Input: dimensioned drawing with shaded views. Units: mm. Origin: part minimum x, y, z. A direction names the side the tool comes from. Round coordinates to 2 decimals unless told otherwise and drop trailing zeros. Order: outer loops, then holes, each group sorted by start corner. A loop starts at its lowest first (then second) coordinate and runs counter-clockwise, first axis right, second up. Notation, with made-up numbers: M 47.5,45 L 98.5,45 A27 ccw 98.5,78 Z; hole C 1,85 d6. An arc over 180 degrees is marked long. Put each result on its own line as item: value. Start each with the question number.
1) Section B-B, the plane y = 0.55. Return loops of the section in (x, z), then the cut area to 3 significant figures.
2) Section C-C, the plane x = 12.25. Return loops of the section in (y, z), then the cut area to 3 significant figures.
3) Section A-A, the plane z = 3.75. Return loops of the section in (x, y).
4) Material intervals for probe 1 along X at (y, z) = (1.2, 4); probe 2 along Z at (x, y) = (5.5, 1.9); probe 3 along X at (y, z) = (2.25, 6.25), sorted ascending. Write a range as [from, to].
5) Section D-D, the plane z = 6.25. Return loops of the section in (x, y), then the cut area to 3 significant figures.
6) Draft query along X for the marked faces 1, 2 and 3. Return one class per face: pulls with the +X half, pulls with the -X half, needs draft (parallel to the pull), parting line crosses it, or undercut.
7) Access query for the marked faces 4 and 5. Directions: +Z, -Z, +X, -X, +Y, -Y. A direction counts if a zero-diameter tool reaches every point of the face in a straight line with its end or side. Return the directions, or none.
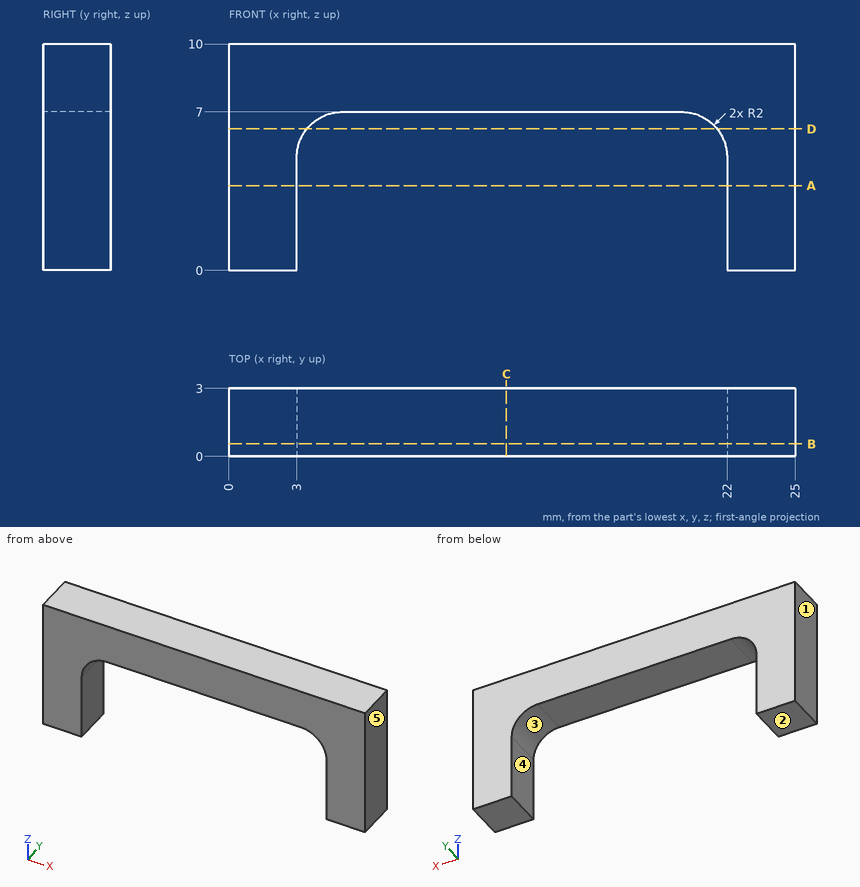
Result sheet:
1. outline: M 0,0 L 3,0 L 3,5 A2 cw 5,7 L 20,7 A2 cw 22,5 L 22,0 L 25,0 L 25,10 L 0,10 Z
1. area: 119 mm2
2. outline: M 0,7 L 3,7 L 3,10 L 0,10 Z
2. area: 9.00 mm2
3. outline: M 0,0 L 3,0 L 3,3 L 0,3 Z; M 22,0 L 25,0 L 25,3 L 22,3 Z
4. probe 1: x = [0, 3], [22, 25]
4. probe 2: z = [7, 10]
4. probe 3: x = [0, 3.44], [21.56, 25]
5. outline: M 0,0 L 3.44,0 L 3.44,3 L 0,3 Z; M 21.56,0 L 25,0 L 25,3 L 21.56,3 Z
5. area: 20.6 mm2
6. face 1: pulls with the -X half
6. face 2: needs draft
6. face 3: undercut
7. face 4: -Z, +Y, -Y
7. face 5: +Z, -Z, +X, +Y, -Y
